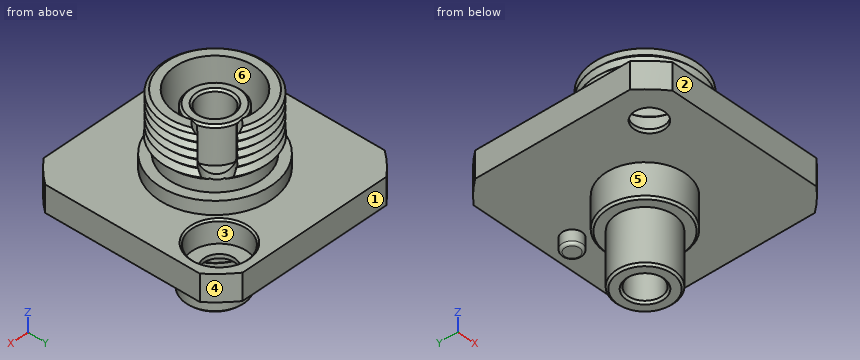
```python
from build123d import *

# Parameters (mm, degrees)
ESQUISSE1_R                                = 3
BOSS_EXTRU_1_DEPTH                         = 2
CHAMBRAGE_POUR_VIS_T_TE_HEXAGONALE_2_COUNT = 2
CHAMBRAGE_POUR_VIS_T_TE_HEXAGONALE_2_PITCH = 13.435028843
CHAMBRAGE_POUR_VIS_T_TE_HEXAGONALE_3_COUNT = 2
CHAMBRAGE_POUR_VIS_T_TE_HEXAGONALE_3_PITCH = 6.717514421
ENL_V_MAT_EXTRU_1_DEPTH                    = 7.3
ESQUISSE10_R                               = 0.75
BOSS_EXTRU_2_DEPTH                         = 1
CONG_1_R                                   = 0.2


with BuildPart() as part:
    # Esquisse1 → Boss.-Extru.1 (new body)
    with BuildSketch(Plane.XY):
        with BuildLine():
            Line((-5.830951895, 7.5), (5.830951895, 7.5))
            ThreePointArc((5.830951895, 7.5), (6.717514421, 6.717514421), (7.5, 5.830951895))
            Line((7.5, 5.830951895), (7.5, -5.830951895))
            ThreePointArc((7.5, -5.830951895), (6.717514421, -6.717514421), (5.830951895, -7.5))
            Line((5.830951895, -7.5), (-5.830951895, -7.5))
            ThreePointArc((-5.830951895, -7.5), (-6.717514421, -6.717514421), (-7.5, -5.830951895))
            Line((-7.5, -5.830951895), (-7.5, 5.830951895))
            ThreePointArc((-7.5, 5.830951895), (-6.717514421, 6.717514421), (-5.830951895, 7.5))
        make_face()
        Circle(ESQUISSE1_R, mode=Mode.SUBTRACT)
    extrude(amount=BOSS_EXTRU_1_DEPTH)

    # Esquisse3 → Révolution1 (revolve)
    with BuildSketch(Plane(origin=(0, 0, 0), x_dir=(0, 0, -1), z_dir=(1, 0, 0)), mode=Mode.PRIVATE) as r_volution1_sk:
        Polygon((-7.5, 3.645251177), (-7.5, 3), (-3.7, 3), (-3.7, 2), (-6.35, 2), (-6.5, 1.85), (-6.5, 1.4), (-6.35, 1.25), (6.4, 1.25), (6.55, 1.4), (6.55, 2.025), (6.4, 2.175), (2.5, 2.175), (2.5, 2.85), (2.35, 3), (-2, 3), (-2, 4.25), (-3, 4.25), (-3, 3.5), (-4, 3.5), (-4, 3.6), (-4.338552793, 3.938552793), (-4.677105586, 3.6), (-4.977105586, 3.9), (-5.277105586, 3.6), (-5.577105586, 3.9), (-5.877105586, 3.6), (-6.177105586, 3.9), (-6.477105586, 3.6), (-6.777105586, 3.9), (-7.077105586, 3.6), (-7.3, 3.9), align=None)
    revolve(r_volution1_sk.sketch.rotate(Axis((0, 0, -5.875), (0, 0, 1)), 90), axis=Axis((0, 0, -5.875), (0, 0, 1)))

    # Esquisse6 → Chambrage pour vis à tête hexagonale M31 (revolve, cut)
    with BuildSketch(Plane(origin=(4.75, 4.75, 2), x_dir=(0, -1, 0), z_dir=(1, 0, 0))):
        Polygon((0, 0), (0, 8.55), (1.15, 8.55), (1.15, 1.7), (2.075, 1.7), (2.075, 0.125), (2.2, 0), align=None)
    chambrage_pour_vis_t_te_hexagonale_m31 = revolve(axis=Axis((4.75, 4.75, 8.35), (0, 0, -1)), mode=Mode.SUBTRACT)

    # Chambrage pour vis _ t_te hexagonale 2: Chambrage pour vis à tête hexagonale M31 ×2
    with Locations(*[Vector(-0.7071067811865475, -0.7071067811865477, 0) * (i * CHAMBRAGE_POUR_VIS_T_TE_HEXAGONALE_2_PITCH) for i in range(1, CHAMBRAGE_POUR_VIS_T_TE_HEXAGONALE_2_COUNT)]):
        add(chambrage_pour_vis_t_te_hexagonale_m31, mode=Mode.SUBTRACT)

    # Chambrage pour vis _ t_te hexagonale 3: Chambrage pour vis à tête hexagonale M31 ×2
    with Locations(*[Vector(-0.7071067811865475, -0.7071067811865477, 0) * (i * CHAMBRAGE_POUR_VIS_T_TE_HEXAGONALE_3_PITCH) for i in range(1, CHAMBRAGE_POUR_VIS_T_TE_HEXAGONALE_3_COUNT)]):
        add(chambrage_pour_vis_t_te_hexagonale_m31, mode=Mode.SUBTRACT)

    # Esquisse9 → Enlèv. mat.-Extru.1 (cut)
    with BuildSketch(Plane(origin=(6.665475947, 6.665475947, 0), x_dir=(-0.7071067811865462, 0.7071067811865488, 0), z_dir=(0.7071067811865488, 0.7071067811865462, 0))):
        with BuildLine():
            Line((1.1, 7.2), (1.1, 5))
            ThreePointArc((1.1, 5), (0, 3.9), (-1.1, 5))
            Line((-1.1, 5), (-1.1, 7.2))
            Line((-1.1, 7.2), (-2.12556829, 8.22556829))
            Line((-2.12556829, 8.22556829), (2.12556829, 8.22556829))
            Line((2.12556829, 8.22556829), (1.1, 7.2))
        make_face()
    extrude(amount=-ENL_V_MAT_EXTRU_1_DEPTH, mode=Mode.SUBTRACT)

    # Esquisse10 → Boss.-Extru.2 (add)
    with BuildSketch(Plane(origin=(0, 0, 0), x_dir=(-1, 0, 0), z_dir=(0, 0, -1))):
        with Locations(Location((0, 5.5, 0), (0, 0, 180))):
            Circle(ESQUISSE10_R)
    extrude(amount=BOSS_EXTRU_2_DEPTH)

    # Congé1
    cong_1_edges = [part.edges().sort_by_distance(p)[0] for p in [
        (-0.75, 5.5, -1),
    ]]
    fillet(cong_1_edges, radius=CONG_1_R)


solid = part.part
```
For this review, take the finished solid that the model builds, in its own axes (mm). Face numbers are marked on the shaded views. A direction names the side the tool comes from. Round coordinates to 2 decimals unless told otherwise and drop trailing zeros. Order: outer loops, then holes, each group sorted by start corner. A loop starts at its lowest first (then second) coordinate and runs counter-clockwise, first axis right, second up.
Q1. Wall thickness on line 1 (X direction, y = 4.75, z = 0.15); line 2 (Z direction, x = -2, y = 1.5); line 3 (Z direction, x = 2, y = 6.5): over which ranges is each line inside the solid? List them lowest first.
Findings below:
line 1: x = -7.5 to 3.6, 5.9 to 7.5
line 2: z = -2.5 to 3.7
line 3: z = 0 to 2
Q2. Insertion check: P1, Ø3.5, axis at x = 4.75, y = 4.75, coming from the +Z side; P2, Ø1, axis at x = -0.5, z = -4, coming from the -Y side (3 decimals); P3, Ø1, axis at x = -0.5, y = -6, coming from the +Z side; P4, Ø3, axis at x = 0, y = 0, coming from the -Z side. Each pin has a flat end and moves straight along its axis. Give the tip position at first contact, or say it passes through.
Findings below:
P1: stops at z = 0.3
P2: stops at y = -2.175
P3: stops at z = 2
P4: stops at z = -6.55
Q3. We need section C-C, the plane z = -3.5. Give the boundary of the cut face in (x, y) (3 decimals).
Findings below:
outline: circle Ø4.35 at (0, 0); hole circle Ø2.5 at (0, 0)
Q4. Machinability: for the marked faces 4, 5 and 6, which of the approach directions +Z, -Z, +X, -X, +Y, -Y give a long, thin tool a straight path to every point of the face, cutting with its end or side? Answer none if there is none.
Findings below:
face 4: +Z, -Z, +X, +Y
face 5: -Z
face 6: +Z
Q5. We need section A-A, the plane y = -4.75. Give the boundary of the cut face in (x, z) (3 decimals).
Findings below:
outline: (-7.5, 0) - (-5.9, 0) - (-5.9, 0.3) - (-6.825, 0.3) - (-6.825, 1.875) - (-6.95, 2) - (-7.5, 2) - close; (-3.6, 0) - (7.5, 0) - (7.5, 2) - (-2.55, 2) - (-2.675, 1.875) - (-2.675, 0.3) - (-3.6, 0.3) - close
Q6. Mouldability with a two-part tool opening along Y and no side actions: class the marked faces 1, 2 and 3 as pulls with the +Y half, pulls with the -Y half, needs draft (parallel to the pull), parting line crosses it, or undercut.
Findings below:
face 1: pulls with the +Y half
face 2: pulls with the -Y half
face 3: undercut
Q7. We need section B-B, the plane z = 1.25. Give the boundary of the cut face in (x, y) (3 decimals).
Findings below:
outline: (-7.5, -5.831) arc R9.5 ccw to (-5.831, -7.5) - (5.831, -7.5) arc R9.5 ccw to (7.5, -5.831) - (7.5, 5.831) arc R9.5 ccw to (5.831, 7.5) - (-5.831, 7.5) arc R9.5 ccw to (-7.5, 5.831) - close; hole circle Ø4.15 at (-4.75, -4.75); hole circle Ø4.15 at (0, 0); hole circle Ø4.15 at (4.75, 4.75)
